from build123d import *

# Parameters (mm, degrees)
SKETCH1_R           = 12.5
BOSS_EXTRUDE1_DEPTH = 40
SKETCH2_R           = 10.02
BOSS_EXTRUDE2_DEPTH = 35
CHAMFER1_SIZE       = 1


with BuildPart() as part:
    # Sketch1 → Boss-Extrude1 (new body)
    with BuildSketch(Plane.XY):
        Circle(SKETCH1_R)
    extrude(amount=-BOSS_EXTRUDE1_DEPTH)

    # Sketch2 → Boss-Extrude2 (add)
    with BuildSketch(Plane(origin=(0, 0, -40), x_dir=(-1, 0, 0), z_dir=(0, 0, -1))):
        Circle(SKETCH2_R)
    extrude(amount=BOSS_EXTRUDE2_DEPTH)

    # Chamfer1
    chamfer1_edges = [part.edges().sort_by_distance(p)[0] for p in [
        (10.02, 0, -75),
    ]]
    chamfer(chamfer1_edges, length=CHAMFER1_SIZE)


solid = part.part
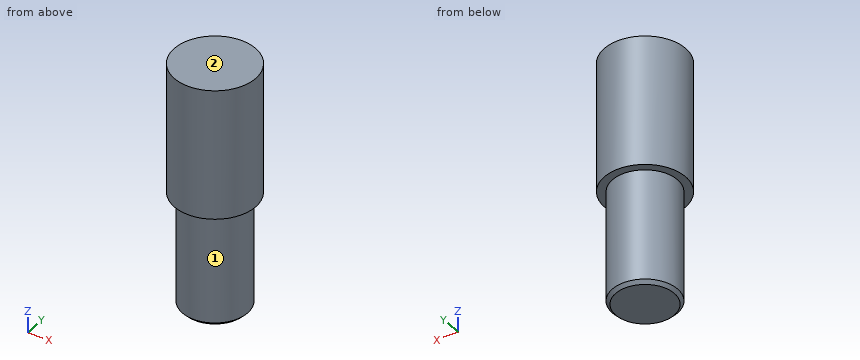
Work out the finished part from the listing and answer in its coordinate system (mm). Face numbers are marked on the shaded views. A direction names the side the tool comes from. Coordinates: 2 decimals unless noted, no trailing zeros. Write each loop counter-clockwise with the first axis right and the second up, starting at its lowest first coordinate (ties: lowest second). Pieces come first, ordered by that corner, then holes.
1. For the marked faces 1 and 2, determine the directions among +Z, -Z, +X, -X, +Y, -Y from which every point of the face is accessible in a straight line to the end or side of a thin tool.
Results list:
face 1: -Z
face 2: +Z, +X, -X, +Y, -Y
2. Consider line 1 along Y through (x, z) = (0.5, -43.5); line 2 along Z through (x, y) = (9.5, -5.5); line 3 along Z through (x, y) = (9, 3.75). Determine where each line is inside the solid, lowest interval first.
Results list:
line 1: y = -10.01 to 10.01
line 2: z = -40 to 0
line 3: z = -74.27 to 0
3. The part is cut by section C-C, the plane z = -28. Write down the section's boundary in (x, y).
Results list:
outline: circle Ø25 at (0, 0)
4. Flat-ended cylindrical pins translate along their axes: pin 1 (10 mm diameter, centred on y = 1.5, z = -20.5, fed in from -X); pin 2 (10 mm diameter, centred on x = 9.5, z = -65, fed in from +Y); pin 3 (5 mm diameter, centred on y = 8, z = -30.5, fed in from -X) (3 decimals); pin 4 (1 mm diameter, centred on x = -6, z = -15, fed in from -Y) (3 decimals). Find the tip coordinate at first contact, or state that the pin passes through.
Results list:
pin 1: stops at x = -12.5
pin 2: stops at y = 8.95
pin 3: stops at x = -11.225
pin 4: stops at y = -11.225
5. The part is cut by section A-A, the plane y = 0. Write down the section's boundary in (x, z).
Results list:
outline: (-12.5, -40) - (-10.02, -40) - (-10.02, -74) - (-9.02, -75) - (9.02, -75) - (10.02, -74) - (10.02, -40) - (12.5, -40) - (12.5, 0) - (-12.5, 0) - close
6. The part is cut by section D-D, the plane z = -69.5. Write down the section's boundary in (x, y), and give its area (3 significant figures).
Results list:
outline: circle Ø20.04 at (0, 0)
area: 315 mm2
